from build123d import *

# Parameters (mm, degrees)
BASPROSKE_W        = 6.35
BASPROSKE_H        = 34.29
TOOTHCUT_DEPTH     = 49.907368565
TEETHCUTS_COUNT    = 25
TEETHCUTS_ANGLE    = 345.6
BORSKE_R           = 6.35
BORE_DEPTH         = 50.8000508
CUT_EXTRUDE1_DEPTH = 3


with BuildPart() as part:
    # BasProSke → Base-Revolve (revolve)
    with BuildSketch(Plane(origin=(0, 0, 0), x_dir=(1, 0, 0), z_dir=(0, 1, 0)), mode=Mode.PRIVATE) as base_revolve_sk:
        with Locations((3.175, 17.145)):
            Rectangle(BASPROSKE_W, BASPROSKE_H)
    revolve(base_revolve_sk.sketch.rotate(Axis((-10, 0, 0), (1, 0, 0)), 180), axis=Axis((-10, 0, 0), (1, 0, 0)))

    # TooCutSke → ToothCut (cut, through all)
    with BuildSketch(Plane(origin=(0, 0, 0), x_dir=(0, 0, -1), z_dir=(1, 0, 0))):
        with BuildLine():
            ThreePointArc((1.227638411, 28.547345762), (0, 28.57373), (-1.227638411, 28.547345762))
            ThreePointArc((-1.227638411, 28.547345762), (-2.085725605, 31.480614743), (-3.619717638, 34.123955242))
            ThreePointArc((-3.619717638, 34.123955242), (0, 34.3154), (3.619717638, 34.123955242))
            ThreePointArc((3.619717638, 34.123955242), (2.085725605, 31.480614743), (1.227638411, 28.547345762))
        make_face()
    toothcut = extrude(amount=TOOTHCUT_DEPTH, mode=Mode.SUBTRACT)

    # TeethCuts: ToothCut ×25 about axis
    teethcuts_axis = Axis((-10, 0, 0), (1, 0, 0))
    for i in range(1, TEETHCUTS_COUNT):
        add(toothcut.rotate(teethcuts_axis, i * TEETHCUTS_ANGLE / (TEETHCUTS_COUNT - 1)), mode=Mode.SUBTRACT)

    # BorSke → Bore (cut, symmetric)
    with BuildSketch(Plane(origin=(0, 0, 0), x_dir=(0, 0, -1), z_dir=(1, 0, 0))):
        with Locations(Location((0, 0, 0), (0, 0, 180))):
            Circle(BORSKE_R)
    extrude(amount=BORE_DEPTH, both=True, mode=Mode.SUBTRACT)

    # Sketch1 → Cut-Extrude1 (cut)
    with BuildSketch(Plane(origin=(6.35, 0, 0), x_dir=(0, 0, -1), z_dir=(1, 0, 0))):
        with BuildLine():
            Line((17.898853189, -2.467978147), (8.419183588, -4))
            Line((8.419183588, -4), (3.919183588, -4))
            add(Edge.make_bspline(
                [(3.919183588, -4), (0, -7.2), (-3.919183588, -4)],
                knots=[0, 0, 0, 1, 1, 1], degree=2))
            Line((-3.919183588, -4), (-8.419183588, -4))
            Line((-8.419183588, -4), (-17.898853189, -2.467978147))
            add(Edge.make_bspline(
                [(-17.898853189, 2.467978147), (-19.149615056, 2.509332033), (-19.873380367, 2.372025905), (-20.078667352, -1.208741201), (-19.543433152, -2.606773936), (-17.898853189, -2.467978147)],
                knots=[0, 0, 0, 0, 0.571712182, 0.671712182, 1, 1, 1, 1], degree=3))
            Line((-17.898853189, 2.467978147), (-8.419183588, 4))
            Line((-8.419183588, 4), (-3.919183588, 4))
            add(Edge.make_bspline(
                [(3.919183588, 4), (0, 7.2), (-3.919183588, 4)],
                knots=[0, 0, 0, 1, 1, 1], degree=2))
            Line((3.919183588, 4), (8.419183588, 4))
            Line((8.419183588, 4), (17.898853189, 2.467978147))
            add(Edge.make_bspline(
                [(17.898853189, 2.467978147), (19.569523565, 2.444629682), (20.025416522, 1.325706455), (19.979573656, -1.037983093), (20.186538624, -2.400122897), (17.898853189, -2.467978147)],
                knots=[0, 0, 0, 0, 0.495063361, 0.595063361, 1, 1, 1, 1], degree=3))
        make_face()
    extrude(amount=-CUT_EXTRUDE1_DEPTH, mode=Mode.SUBTRACT)


solid = part.part
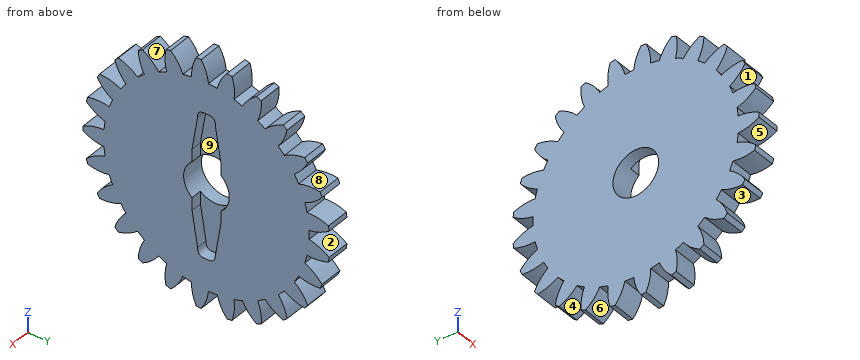
For this review, take the finished solid that the model builds, in its own axes (mm). Face numbers are marked on the shaded views. A direction names the side the tool comes from. Give positions to 0.01 mm unless a question says otherwise; leave off trailing zeros. Loops run counter-clockwise (first coordinate to the right, second up) from the corner with the lowest first, then second, coordinate; pieces in that order, holes last.
Item 1: Take a section at B-B, the plane y = 12.5. State the section outline as (x, z) points.
Item 2: For line 1 along Y through (x, z) = (4.5, 0); line 2 along Y through (x, z) = (4.25, 19); line 3 along Z through (x, y) = (0.5, -24), list the stretches that pass through material, from the lowest coordinate up.
Item 3: Insertion check: pin 1 (3 mm diameter, centred on x = 5.5, z = 24, fed in from +Y); pin 2 (4 mm diameter, centred on y = 0.5, z = 15.5, fed in from +X); pin 3 (7.5 mm diameter, centred on y = 0, z = 0, fed in from +X); pin 4 (2.5 mm diameter, centred on x = 5, z = -7, fed in from -Y). Each pin has a flat end and moves straight along its axis. Give the tip position at first contact, or say it passes through.
Item 4: Tool access review of the marked faces 5, 6, 7, 8 and 9: name each direction out of +Z, -Z, +X, -X, +Y, -Y from which nothing blocks a thin tool from reaching the whole face with its end or side.
Item 5: Take a section at A-A, the plane y = -20. State the section outline as (x, z) points.
Item 6: Draft analysis for pull direction Y (two halves, no side actions). For the marked faces 1, 2, 3 and 4, state which applies: +Y half, -Y half, draft (parallel to the pull), parting line (faces both ways), or undercut.
Calculated:
1. outline: (0, -30.12) - (6.35, -30.12) - (6.35, 30.12) - (0, 30.12) - close
2. line 1: y = -34.29 to -6.35, 6.35 to 28.57
2. line 2: y = -23.44 to -2.33, 2.39 to 21.34, 22.21 to 27.87
2. line 3: z = -23.84 to -19.8, -15.88 to 15.88, 19.8 to 23.84
3. pin 1: stops at y = 22.3
3. pin 2: stops at x = 3.35
3. pin 3: passes through
3. pin 4: stops at y = -33.38
4. face 5: +X, -X, -Y
4. face 6: -Z, +X, -X
4. face 7: +Z, +X, -X
4. face 8: +X, -X
4. face 9: +X
5. outline: (0, -21.9) - (6.35, -21.9) - (6.35, 21.9) - (0, 21.9) - close
6. face 1: -Y half
6. face 2: +Y half
6. face 3: undercut
6. face 4: undercut
